from build123d import *

# Parameters (mm, degrees)
BOSS_EXTRU_1_DEPTH                = 50
COQUE2_T                          = -10
TROU_TARAUD_0_801_D               = 12
TROU_DE_PASSAGE_D_AXE_3_321_D     = 8.0000094
TROU_DE_PASSAGE_D_AXE_3_321_DEPTH = 10


with BuildPart() as part:
    # Esquisse1 → Boss.-Extru.1 (new body)
    with BuildSketch(Plane.XY):
        with BuildLine():
            Line((0, 0), (0, 68))
            Line((0, 68), (44.704064579, 68))
            ThreePointArc((44.704064579, 68), (37.345127658, 33.967330015), (45, 0))
            Line((45, 0), (0, 0))
        make_face()
    extrude(amount=BOSS_EXTRU_1_DEPTH)

    # Coque2
    coque2_openings = [part.faces().sort_by_distance(p)[0] for p in [
        (19.961549488, 33.959529951, 0),
    ]]
    offset(amount=COQUE2_T, openings=coque2_openings, kind=Kind.INTERSECTION)

    # Trou taraudé #0-801 (through all)
    with Locations(Plane.XY.offset(50)):
        with Locations((20.726437539, 25)):
            Hole(TROU_TARAUD_0_801_D / 2)

    # Trou de passage d'axe 3/321
    with Locations(Plane(origin=(37.374610437, 32.108761201, 28.657882027), x_dir=(-0.027368282342, 0.999625418405, 0), z_dir=(0.999625418405, 0.027368282342, 0))):
        with Locations((0, 0)):
            Hole(TROU_DE_PASSAGE_D_AXE_3_321_D / 2, depth=TROU_DE_PASSAGE_D_AXE_3_321_DEPTH)


solid = part.part
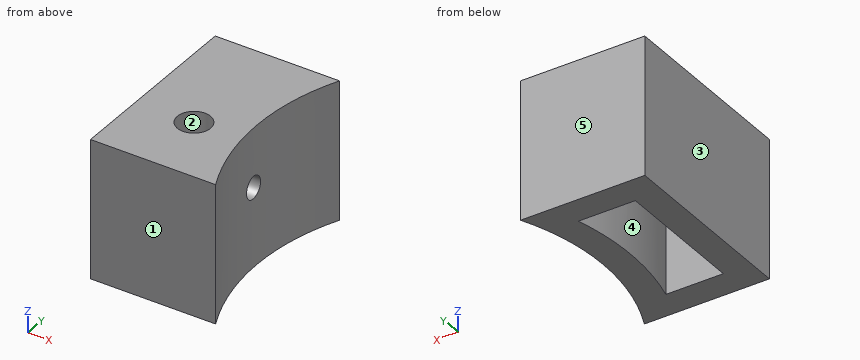
Read the model definition and answer for the solid it produces. Units are mm, in the model's axes. Face numbers are marked on the shaded views. A direction names the side the tool comes from. Round coordinates to 2 decimals unless told otherwise and drop trailing zeros. Loops run counter-clockwise (first coordinate to the right, second up) from the corner with the lowest first, then second, coordinate; pieces in that order, holes last. Notation, with made-up numbers: (5.5, 45) - (44.5, 45) arc R11 cw to (44.5, 49) - close; hole circle Ø4 at (75.5, 85.25). An arc over 180 degrees is marked (long way). One line per question, with ' | ' between items. Start each with the question number.
Q1. For the marked faces 4 and 5, determine the directions among +Z, -Z, +X, -X, +Y, -Y from which every point of the face is accessible in a straight line to the end or side of a thin tool.
Q2. Section D-D on y = 45 is taken. Give the vertices of the cut face in (x, z).
Q3. Section B-B on y = 25 is taken. Give the vertices of the cut face in (x, z), plus the area to 3 significant figures.
Q4. For a pull along Y with two mould halves and no side action, classify the marked faces 1, 2 and 3 as +Y half, -Y half, draft (parallel to the pull), parting line (faces both ways), or undercut.
Q5. Section C-C on x = 21 is taken. Give the vertices of the cut face in (y, z), plus the area to 3 significant figures.
Q6. Flat-ended cylindrical pins translate along their axes: pin 1 (19 mm diameter, centred on x = 20.73, y = 25, fed in from +Z); pin 2 (5 mm diameter, centred on y = 27, z = 13, fed in from +X); pin 3 (6 mm diameter, centred on y = 46.5, z = 25.5, fed in from +X); pin 4 (4 mm diameter, centred on y = 37.5, z = 12, fed in from +X). Find the tip coordinate at first contact, or state that the pin passes through.
Q7. Find the intervals of material crossed by L1, parallel to Y at x = 25.5, z = 9; L2, parallel to X at y = 22, z = 14.5; L3, parallel to Z at x = 28, y = 13, in increasing order.
Q8. Section A-A on z = 8 is taken. Give the vertices of the cut face in (x, y).
Established:
1) face 4: -Z | face 5: +Z, -Z, +X, -X, +Y
2) outline: (0, 0) - (10, 0) - (10, 40) - (27.98, 40) - (27.98, 0) - (38.05, 0) - (38.05, 50) - (0, 50) - close
3) outline: (0, 0) - (10, 0) - (10, 40) - (14.73, 40) - (14.73, 50) - (0, 50) - close; (26.73, 40) - (27.82, 40) - (27.82, 0) - (37.88, 0) - (37.88, 50) - (26.73, 50) - close | area: 1,060 mm²
4) face 1: -Y half | face 2: undercut | face 3: draft
5) outline: (0, 0) - (10, 0) - (10, 40) - (19.01, 40) - (19.01, 50) - (0, 50) - close; (30.99, 40) - (58, 40) - (58, 0) - (68, 0) - (68, 50) - (30.99, 50) - close | area: 1,360 mm²
6) pin 1: z = 50 | pin 2: x = 37.94 | pin 3: x = 38.78 | pin 4: x = 37.51
7) L1: 0 to 10, 58 to 68 | L2: 0 to 10, 28.18 to 38.29 | L3: 40 to 50
8) outline: (0, 0) - (45, 0) arc R80.75 cw to (44.7, 68) - (0, 68) - close; hole (10, 10) - (30.66, 10) arc R90.75 cw to (30.49, 58) - (10, 58) - close
